Can you work these out from the drawing? Everything is in mm from the part's minimum corner. A direction names the side the tool comes from. Round coordinates to 2 decimals unless told otherwise and drop trailing zeros. Write each loop counter-clockwise with the first axis right and the second up, starting at its lowest first coordinate (ties: lowest second). Pieces come first, ordered by that corner, then holes. Notation, with made-up numbers: (-15, -40) - (2, -40) arc R24 cw to (2, -16) - close; hole circle Ø8 at (35.25, -39.75). An arc over 180 degrees is marked (long way). One line per item, written item: value. Start each with the question number.
Item 1: For the marked faces 1 and 2, which set-ups out of +Z, -Z, +X, -X, +Y, -Y let a thin tool reach every point of the face, with its end or its side?
Item 2: If I drill on line 1 (X direction, y = 0.75, z = 26); line 2 (Z direction, x = 0.3, y = 14); line 3 (Y direction, x = 11.5, z = 29), over which ranges is the centre line in solid material (lowest first)?
Item 3: For P1, Ø12, axis at y = 13, z = 12, coming from the +X side, with a flat end and sliding along its axis, tell me the tip position at first contact or that it passes through.
Item 4: Imagine slicing it at C-C, the plane z = 26. Please give me the cut outline in (x, y).
Item 5: Imagine slicing it at D-D, the plane z = 12. Please give me the cut outline in (x, y).
Item 6: Imagine slicing it at B-B, the plane x = 11.25. Please give me the cut outline in (y, z), then the cut area to 3 significant figures.
Item 7: Imagine slicing it at A-A, the plane y = 15.25. Please give me the cut outline in (x, z).
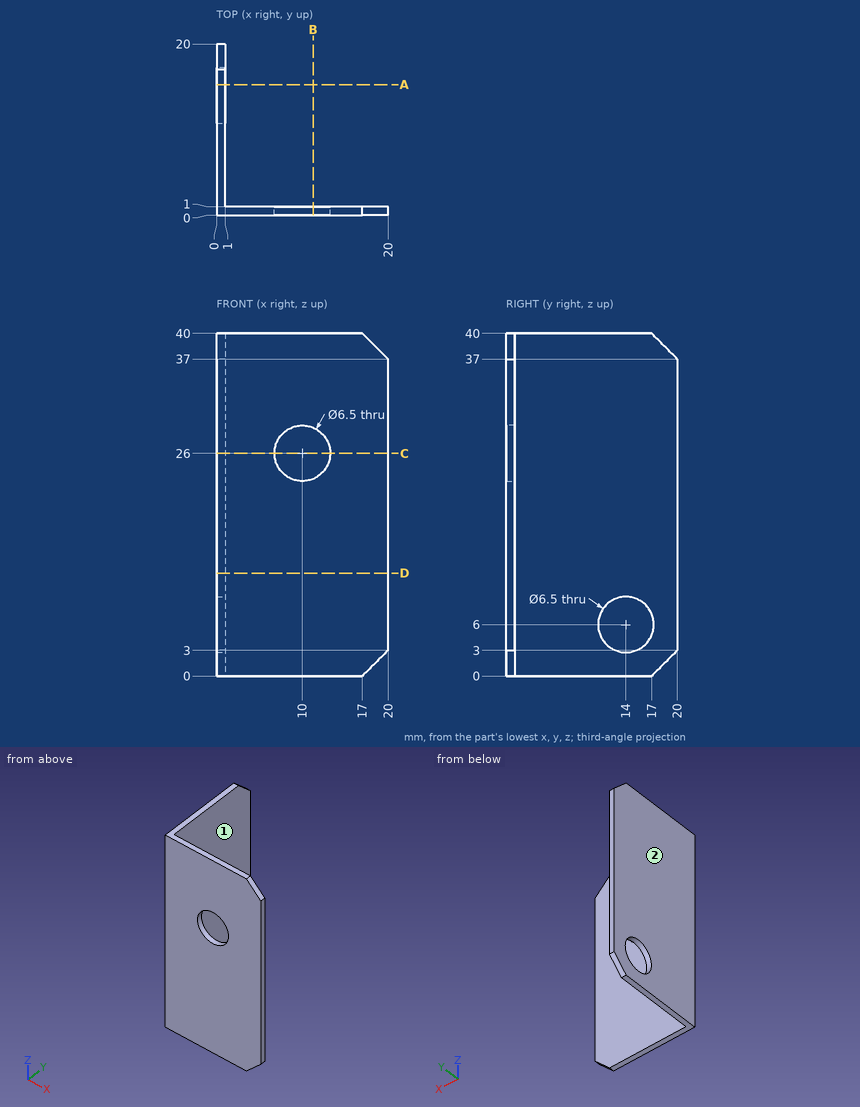
Values follow:
1. face 1: +Z, -Z, +X, +Y
1. face 2: +Z, -Z, -X, +Y, -Y
2. line 1: x = 0 to 6.75, 13.25 to 20
2. line 2: z = 0 to 2.75, 9.25 to 40
2. line 3: y = 0 to 1
3. P1: stops at x = 1
4. outline: (0, 0) - (6.75, 0) - (6.75, 1) - (1, 1) - (1, 20) - (0, 20) - close; (13.25, 0) - (20, 0) - (20, 1) - (13.25, 1) - close
5. outline: (0, 0) - (20, 0) - (20, 1) - (1, 1) - (1, 20) - (0, 20) - close
6. outline: (0, 0) - (1, 0) - (1, 23) - (0, 23) - close; (0, 29) - (1, 29) - (1, 40) - (0, 40) - close
6. area: 34.0 mm^2
7. outline: (0, 0) - (1, 0) - (1, 3) - (0, 3) - close; (0, 9) - (1, 9) - (1, 40) - (0, 40) - close
